Can you work these out from the model? Positions are in its coordinate system, mm. A direction names the side the tool comes from. Coordinates: 2 decimals unless noted, no trailing zeros. Order: outer loops, then holes, each group sorted by start corner. A loop starts at its lowest first (then second) coordinate and runs counter-clockwise, first axis right, second up.
```python
from build123d import *

# Parameters (mm, degrees)
BOSS_EXTRUDE2_DEPTH = 6.35
SKETCH4_R           = 3.175
CUT_EXTRUDE1_DEPTH  = 12.7
CUT_EXTRUDE2_DEPTH  = 2.032


with BuildPart() as part:
    # Sketch3 → Boss-Extrude2 (new body)
    with BuildSketch(Plane(origin=(0, 0, 0), x_dir=(1, 0, 0), z_dir=(0, 1, 0))):
        with BuildLine():
            Line((-19.05, 5.08), (19.05, 5.08))
            ThreePointArc((19.05, 5.08), (19.715701864, 0), (19.05, -5.08))
            Line((19.05, -5.08), (-19.05, -5.08))
            ThreePointArc((-19.05, -5.08), (-19.715701864, 0), (-19.05, 5.08))
        make_face()
    extrude(amount=BOSS_EXTRUDE2_DEPTH)

    # Sketch4 → Cut-Extrude1 (cut)
    with BuildSketch(Plane(origin=(0, 6.35, 0), x_dir=(1, 0, 0), z_dir=(0, 1, 0))):
        with Locations((15.24, 0)):
            Circle(SKETCH4_R)
        with Locations((-15.24, 0)):
            Circle(SKETCH4_R)
    extrude(amount=-CUT_EXTRUDE1_DEPTH, mode=Mode.SUBTRACT)

    # Sketch5 → Cut-Extrude2 (cut)
    with BuildSketch(Plane.XZ):
        with BuildLine():
            Line((19.05, 5.08), (-2.54, 5.08))
            Line((-2.54, 5.08), (-2.54, -5.08))
            Line((-2.54, -5.08), (19.05, -5.08))
            ThreePointArc((19.05, -5.08), (19.715701864, 0), (19.05, 5.08))
        make_face()
    extrude(amount=-CUT_EXTRUDE2_DEPTH, mode=Mode.SUBTRACT)


solid = part.part
```
1. On a 3-axis mill with a long thin cutter (end or side, diameter ignored), from which of +Z, -Z, +X, -X, +Y, -Y can I reach the whole of each face in a straight line? I mean faces 1 (the cylindrical face through (19.716, 4.161, -0.072)), 2 (the flat face through (8, 2.032, 0)). Say none if no direction works.
Completed:
face 1: +X, +Y, -Y
face 2: +Z, -Z, +X, -Y
2. Imagine slicing it at D-D on x = 15.24. Please give me the cut outline in (y, z) (3 decimals), then the cut area to 3 significant figures.
Completed:
outline: (2.032, -5.08) - (6.35, -5.08) - (6.35, -3.175) - (2.032, -3.175) - close; (2.032, 3.175) - (6.35, 3.175) - (6.35, 5.08) - (2.032, 5.08) - close
area: 16.5 mm2
3. Imagine slicing it at B-B on z = 0. Please give me the cut outline in (x, y) (3 decimals).
Completed:
outline: (-19.716, 0) - (-18.415, 0) - (-18.415, 6.35) - (-19.716, 6.35) - close; (-12.065, 0) - (-2.54, 0) - (-2.54, 2.032) - (12.065, 2.032) - (12.065, 6.35) - (-12.065, 6.35) - close; (18.415, 2.032) - (19.716, 2.032) - (19.716, 6.35) - (18.415, 6.35) - close
4. Please list where these lines run through material, in increasing order: probe 1 along Z at (x, y) = (15.24, 5.1) (3 decimals); probe 2 along Z at (x, y) = (-14.5, 2.5); probe 3 along X at (y, z) = (0.75, -1).
Completed:
probe 1: z = -5.08 to -3.175, 3.175 to 5.08
probe 2: z = -5.08 to -3.09, 3.09 to 5.08
probe 3: x = -19.69 to -18.25, -12.23 to -2.54
5. Imagine slicing it at C-C on y = 3. Please give me the cut outline in (x, z) (3 decimals).
Completed:
outline: (-19.05, -5.08) - (19.05, -5.08) arc R19.716 ccw to (19.05, 5.08) - (-19.05, 5.08) arc R19.716 ccw to start; hole circle Ø6.35 at (-15.24, 0); hole circle Ø6.35 at (15.24, 0)
6. Imagine slicing it at A-A on x = -15.24. Please give me the cut outline in (y, z) (3 decimals).
Completed:
outline: (0, -5.08) - (6.35, -5.08) - (6.35, -3.175) - (0, -3.175) - close; (0, 3.175) - (6.35, 3.175) - (6.35, 5.08) - (0, 5.08) - close
7. Thinking about a two-plate mould opening in Z: for faces 3 (the flat face through (0, 4, -5.08)), 4 (the cylindrical face through (-19.716, 3.131, 0.072)), 5 (the cylindrical face through (-17.58, 3.219, -2.146)), 6 (the flat face through (0, 4, 5.08)), which applies, pulls with the +Z half, pulls with the -Z half, needs draft (parallel to the pull), parting line crosses it, or undercut?
Completed:
face 3: pulls with the -Z half
face 4: parting line crosses it
face 5: undercut
face 6: pulls with the +Z half
8. I'm going to push flat-ended pins straight in: pin 1 (1 mm diameter, centred on y = 1, z = 0, fed in from +X); pin 2 (3 mm diameter, centred on x = 12, z = -0.5, fed in from -Y); pin 3 (2 mm diameter, centred on y = 2, z = 2, fed in from -X). Where does each tip first touch, or does it pass through?
Completed:
pin 1: stops at x = -2.54
pin 2: stops at y = 2.03
pin 3: stops at x = -19.69
